The model under review builds one solid part; all positions refer to its coordinate system, in mm. Face numbers are marked on the shaded views. A direction names the side the tool comes from. Coordinates: 2 decimals unless noted, no trailing zeros. Loops run counter-clockwise (first coordinate to the right, second up) from the corner with the lowest first, then second, coordinate; pieces in that order, holes last. Notation, with made-up numbers: (71.25, 62.25) - (121.25, 62.25) arc R24 cw to (121.25, 91.25) - close; hole circle Ø7 at (47.5, 59). An arc over 180 degrees is marked (long way). Use a Markdown table: item, result. Add a question column.
1) Add section A-A, the plane z = 0. Give the boundary of the cut face in (x, y).
2) Add section C-C, the plane z = 13. Give the boundary of the cut face in (x, y).
3) For the marked faces 1 and 2, list the 3-axis set-ups (+Z, -Z, +X, -X, +Y, -Y) from which the entire face can be reached by the end or side of a thin tool; tool diameter is ignored.
4) Add section D-D, the plane x = 1.5. Give the boundary of the cut face in (y, z).
5) Add section B-B, the plane y = 16. Give the boundary of the cut face in (x, z).
6) Clearance check with flat-ended pins moving along their axes: pin 1 (3 mm diameter, centred on x = 3, z = 9, fed in from +Y); pin 2 (4 mm diameter, centred on x = 2, z = 13, fed in from +Y). State where each tip first meets the part, or that it passes through.
7) The part is to be moulded in two halves that separate along X. For the marked faces 3, 4 and 5, say which applies: pulls with the +X half, pulls with the -X half, needs draft (parallel to the pull), parting line crosses it, or undercut.
8) To check wall thickness, follow L1, parallel to Z at x = 2, y = 1.45; L2, parallel to X at y = 37, z = -14; L3, parallel to Z at x = 2, y = 4. State the ranges of each line that lie inside material, in increasing order. Write a range as [from, to].
```python
from build123d import *

# Parameters (mm, degrees)
SKETCH1_W                                    = 30
SKETCH1_H                                    = 40
BOSS_EXTRUDE1_DEPTH                          = 45
SKETCH2_W                                    = 10
SKETCH2_H                                    = 40
CUT_EXTRUDE1_DEPTH                           = 63.04836823
SKETCH3_R                                    = 3.5
CUT_EXTRUDE2_DEPTH                           = 58.662812973
CUT_EXTRUDE3_DEPTH                           = 58.662812973
CBORE_FOR_M2_HEX_HEAD_CAP_SCREW1_D           = 2.4
CBORE_FOR_M2_HEX_HEAD_CAP_SCREW1_CBORE_D     = 7.619
CBORE_FOR_M2_HEX_HEAD_CAP_SCREW1_CBORE_DEPTH = 1.4


with BuildPart() as part:
    # Sketch1 → Boss-Extrude1 (new body)
    with BuildSketch(Plane(origin=(0, 0, 0), x_dir=(1, 0, 0), z_dir=(0, 1, 0))):
        Rectangle(SKETCH1_W, SKETCH1_H)
    extrude(amount=BOSS_EXTRUDE1_DEPTH)

    # Sketch2 → Cut-Extrude1 (cut, through all)
    with BuildSketch(Plane.XY.offset(20)):
        with Locations((2, 25)):
            Rectangle(SKETCH2_W, SKETCH2_H)
    extrude(amount=-CUT_EXTRUDE1_DEPTH, mode=Mode.SUBTRACT)

    # Sketch3 → Cut-Extrude2 (cut, through all)
    with BuildSketch(Plane.ZY.offset(15)):
        with Locations((0, 27.391853945)):
            Circle(SKETCH3_R)
    extrude(amount=-CUT_EXTRUDE2_DEPTH, mode=Mode.SUBTRACT)

    # Sketch4 → Cut-Extrude3 (cut, through all)
    with BuildSketch(Plane.ZY.offset(15)):
        with BuildLine():
            Line((-20, 45), (-15, 45))
            ThreePointArc((-15, 45), (-18.535533906, 43.535533906), (-20, 40))
            Line((-20, 40), (-20, 45))
        make_face()
        with BuildLine():
            Line((15, 45), (20, 45))
            Line((20, 45), (20, 40))
            ThreePointArc((20, 40), (18.535533906, 43.535533906), (15, 45))
        make_face()
    extrude(amount=-CUT_EXTRUDE3_DEPTH, mode=Mode.SUBTRACT)

    # CBORE for M2 Hex Head Cap Screw1 (through all)
    with Locations(Plane(origin=(0, 5, 0), x_dir=(1, 0, 0), z_dir=(0, 1, 0))):
        with Locations((2, -13), (2, 13)):
            CounterBoreHole(CBORE_FOR_M2_HEX_HEAD_CAP_SCREW1_D / 2, CBORE_FOR_M2_HEX_HEAD_CAP_SCREW1_CBORE_D / 2, CBORE_FOR_M2_HEX_HEAD_CAP_SCREW1_CBORE_DEPTH)


solid = part.part
```
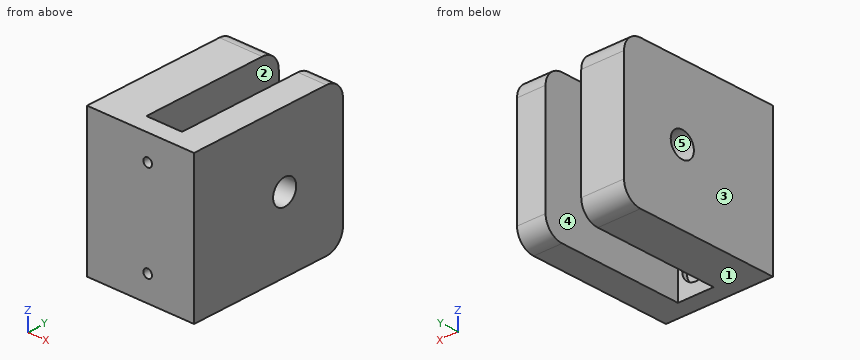
From the geometry:
| question | item | result |
|---|---|---|
| 1 | outline | (-15, 0) - (15, 0) - (15, 23.89) - (7, 23.89) - (7, 5) - (-3, 5) - (-3, 23.89) - (-15, 23.89) - close; (-15, 30.89) - (-3, 30.89) - (-3, 45) - (-15, 45) - close; (7, 30.89) - (15, 30.89) - (15, 45) - (7, 45) - close |
| 2 | outline | (-15, 0) - (0.8, 0) - (0.8, 3.6) - (-1.81, 3.6) - (-1.81, 5) - (-3, 5) - (-3, 45) - (-15, 45) - close; (3.2, 0) - (15, 0) - (15, 45) - (7, 45) - (7, 5) - (5.81, 5) - (5.81, 3.6) - (3.2, 3.6) - close |
| 3 | face 1 | -Z, +X, -X, +Y, -Y |
| 3 | face 2 | +Z, -Z, +Y |
| 4 | outline | (0, -20) - (5, -20) - (5, -16.78) - (3.6, -16.78) - (3.6, -14.09) - (0, -14.09) - close; (0, -11.91) - (3.6, -11.91) - (3.6, -9.22) - (5, -9.22) - (5, 9.22) - (3.6, 9.22) - (3.6, 11.91) - (0, 11.91) - close; (0, 14.09) - (3.6, 14.09) - (3.6, 16.78) - (5, 16.78) - (5, 20) - (0, 20) - close |
| 5 | outline | (-15, -20) - (-3, -20) - (-3, 20) - (-15, 20) - close; (7, -20) - (15, -20) - (15, 20) - (7, 20) - close |
| 6 | pin 1 | stops at y = 5 |
| 6 | pin 2 | stops at y = 3.6 |
| 7 | face 3 | pulls with the -X half |
| 7 | face 4 | undercut |
| 7 | face 5 | needs draft |
| 8 | L1 | z = [-20, -14.2], [-11.8, 11.8], [14.2, 20] |
| 8 | L2 | x = [-15, -3], [7, 15] |
| 8 | L3 | z = [-20, -16.81], [-9.19, 9.19], [16.81, 20] |
